Can you work these out from the model? Positions are in its coordinate system, mm. A direction names the side the tool comes from. Round coordinates to 2 decimals unless told otherwise and drop trailing zeros. Order: outer loops, then holes, each group sorted by start corner. A loop starts at its lowest first (then second) coordinate and runs counter-clockwise, first axis right, second up.
Q1. If we section it at A-A (y = -80): Please give me the cut outline in (x, z), plus the area to 3 significant figures.
Q2. Will these pins go through, and if not, where does the flat tip stop? P1, Ø1.5, axis at x = 105.5, y = -80, coming from the +Z side; P2, Ø22.5, axis at x = 111.47, y = -100.37, coming from the +Z side; P3, Ø3, axis at y = -125.5, z = -17.5, coming from the -X side; P4, Ø1, axis at x = 84, z = -11.5, coming from the -Y side.
Q3. If we section it at B-B (x = 172): Please give me the cut outline in (y, z), plus the area to 3 significant figures.
Q4. If I drill on line 1 (X direction, y = -142, z = -20); line 2 (X direction, y = -26, z = -14.75); line 3 (X direction, y = -155, z = -11.25), over which ranges is the centre line in solid material (lowest first)?
Q5. We'd pull the mould along Z, two halves only. Please class faces 4 (the face through (-142, -29, -12)), 5 (the face through (178.42, -15.21, -12.65)), 6 (the face through (165, 0, -11)): pulls with the +Z half, pulls with the -Z half, needs draft (parallel to the pull), parting line crosses it, or undercut.
Q6. For faces 1 (the face through (-3.316, -169.968, -10.846)), 2 (the face through (180, -30, -6)), 3 (the face through (147, -20, -12)), which set-ups out of +Z, -Z, +X, -X, +Y, -Y let a thin tool reach every point of the face, with its end or its side?
Q7. If we section it at C-C (x = 0): Please give me the cut outline in (y, z), plus the area to 3 significant figures.
Autodesk Inventor part; units mm, degrees
ref_plane "YZ Plane" through (0, 0, 0) normal (1, 0, 0) x (0, 1, 0)
ref_plane "XZ Plane" through (0, 0, 0) normal (0, 1, 0) x (-1, 0, 0)
ref_plane "XY Plane" through (0, 0, 0) normal (0, 0, 1) x (1, 0, 0)
sketch "Sketch1" plane through (0, 0, 0) normal (0, 0, 1) x (1, 0, 0)
  circle A0 centre (0, 0) radius 150 construction
  line L0 (0, 150) -> (0, 170) construction
  line L1 (0, 150) -> (0, 130) construction
  circle A1 centre (0, 0) radius 130
  circle A2 centre (0, 0) radius 170
  line L2 (-130, 0) -> (-130, 80) construction
  line L3 (-130, 80) -> (-170, 80) construction
  line L4 (-170, 80) -> (-170, 0) construction
  line L5 (-130, 0) -> (-170, 0)
  line L6 (-170, 0) -> (-200, 0)
  line L7 (-200, 0) -> (-200, -30)
  line L8 (-200, -30) -> (-167.332, -30)
  line L9 (-1.5, -168) -> (1.5, -168)
  line L10 (1.5, -168) -> (1.5, -210)
  line L11 (1.5, -210) -> (-1.5, -210)
  line L12 (-1.5, -210) -> (-1.5, -168)
  line L13 (0, -168) -> (0, -130)
  line L14 (-1.5, -210) -> (-30, -210)
  line L15 (-30, -210) -> (-30, -167.332)
  line L16 (0, -168) -> (0, -170)
  point P0 (170, 0)
  point P1 (0, -210)
  point P2 (-1.5, -169.9934)
  point P3 (1.5, -169.9934)
  dimension "d26" = 80
  dimension "d36" = 40
  dimension "d40" = 30
  dimension "d41" = 30
  dimension "d74" = 260
  dimension "d75" = 3
  dimension "d76" = 42
  dimension "d77" = 30
  dimension "d78" = 2
extrude "Extrusion1" add sketch "Sketch1" against normal blind 22 contours A1 L13 L9 L12 A2 L5 | A2 L8 L7 L6 | L16 A2 L12 L9
sketch "Sketch10" plane through (-200, -30, 0) normal (0, -1, 0) x (1, 0, 0)
  line L0 (0, 0) -> (32.668, 0)
  line L1 (0, 0) -> (0, -22)
  line L2 (32.668, -22) -> (0, -22)
  line L3 (32.668, 0) -> (32.668, -22)
  circle A0 centre (16.334, -11) radius 5.5
  line L4 (0, 0) -> (0, -22)
  line L5 (0, 0) -> (32.668, 0)
  point P0 (200, 0)
  point P1 (0, -11)
  point P2 (16.334, 0)
  dimension "d79" = 11
extrude "Extrusion9" cut sketch "Sketch10" against normal through all contours A0
mirror "Mirror3" about plane through (0, 0, 0) normal (1, 0, 0) of "Extrusion1", "Extrusion9"
sketch "Sketch12" plane through (0, 0, 0) normal (0, 0, 1) x (1, 0, 0)
  line L0 (0, 0) -> (-150, 0) construction
  line L1 (0, 0) -> (-147.7212, -26.0472) construction
  circle A0 centre (0, 0) radius 150 construction
  dimension "d86" = 10
  dimension "d87" = 300
hole "Hole4" at (-147.7212, -26.0472, 0) direction (0, 0, -1) diameter 11 end through all counterbore diameter 25 counterbore depth 12
pattern_circular "Circular Pattern5" count 6 over 160 about axis through (0, 0, -10) along (0, 0, 1) of "Hole4"
equation "\"d41\" = d40"
equation "\"d93\" = Thickness"
equation "\"BendReliefDepth\" = 0.5 * Thickness"
properties part number "ДМФ 093 Постель КОРМА v2.0" material "Nylon 6"
Solution:
1. outline: (-150, -22) - (-102.47, -22) - (-102.47, 0) - (-150, 0) - close; (102.47, -22) - (150, -22) - (150, 0) - (102.47, 0) - close
1. area: 2,090 mm2
2. P1: stops at z = 0
2. P2: stops at z = -12
2. P3: stops at x = -116.29
2. P4: stops at y = -148.08
3. outline: (-30, -22) - (0, -22) - (0, 0) - (-30, 0) - close
3. area: 660 mm2
4. line 1: x = -93.47 to -46.39, -36.3 to 36.3, 46.39 to 93.47
4. line 2: x = -200 to -187.69, -179.64 to -153.22, -142.22 to -127.37, 127.37 to 142.22, 153.22 to 179.64, 187.69 to 200
4. line 3: x = -69.82 to -47.62, -35.07 to 35.07, 47.62 to 69.82
5. face 4: pulls with the +Z half
5. face 5: undercut
5. face 6: needs draft
6. face 1: +Z, -Z, -Y
6. face 2: +Z, -Z, +X, -Y
6. face 3: +Z
7. outline: (-170, -22) - (-130, -22) - (-130, 0) - (-170, 0) - close
7. area: 880 mm2
